Here's how the part is built. I have some questions about the finished solid (model axes, mm). A direction names the side the tool comes from. Coordinates: 2 decimals unless noted, no trailing zeros. Order: outer loops, then holes, each group sorted by start corner. A loop starts at its lowest first (then second) coordinate and runs counter-clockwise, first axis right, second up. Notation, with made-up numbers: (-39, 28.25) - (-19, 28.25) arc R22 cw to (-19, 46.25) - close; hole circle Ø3 at (-30.5, 21). An arc over 180 degrees is marked (long way). Answer as CSV lines item,"result". Start each with the question number.
Q1. For faces 4 (the face through (-1115, 734, -1921.897)), 5 (the face through (-1143, 746, -1943.397)), 6 (the face through (-1127.528, 743, -1930)), 7 (the face through (-1143, 740, -1917.397)), which set-ups out of +Z, -Z, +X, -X, +Y, -Y let a thin tool reach every point of the face, with its end or its side?
Q2. Thinking about a two-plate mould opening in X: for faces 1 (the face through (-1158.528, 746, -1930)), 2 (the face through (-1128, 732.908, -1929)), 3 (the face through (-1115, 734, -1936.897)), which applies, released by +X, released by -X, zero draft, split by the parting line, or undercut?
Q3. I need wall thicknesses on line 1 (X direction, y = 733.75, z = -1941.5); line 2 (X direction, y = 738.75, z = -1931); line 3 (Z direction, x = -1148.5, y = 729). Which ranges of each line are inside material? Lowest first, please.
Q4. Suppose I cut it at A-A (z = -1926.5). Please give me the cut outline in (x, y), then the cut area to 3 significant figures.
Q5. For pin 1 Ø10 at (y, z) = (731.5, -1931) entering from +X; pin 2 Ø13 at (y, z) = (746.5, -1933) entering from +X; pin 3 Ø4 at (x, y) = (-1151, 737) entering from +Z, each with a flat end and sliding along its axis, tell me the tip position at first contact or that it passes through.
Q6. Suppose I cut it at D-D (x = -1152.5). Please give me the cut outline in (y, z).
Q7. Suppose I cut it at B-B (x = -1121). Please give me the cut outline in (y, z).
Q8. Suppose I cut it at C-C (y = 736.5). Please give me the cut outline in (x, z), then the cut area to 3 significant figures.
from build123d import *

# Parameters (mm, degrees)
SKETCH3_W           = 4000
SKETCH3_H           = 4000
BOSS_EXTRUDE1_DEPTH = 1250
SKETCH4_W           = 3200
SKETCH4_H           = 2700
BOSS_EXTRUDE2_DEPTH = 1200
SKETCH6_W           = 3000
SKETCH6_H           = 2500
CUT_EXTRUDE1_DEPTH  = 6011.745093863
SKETCH9_W           = 2000
SKETCH9_H           = 690
BOSS_EXTRUDE8_DEPTH = 150
SKETCH8_W           = 2000
SKETCH8_H           = 690
BOSS_EXTRUDE9_DEPTH = 150
SKETCH13_W          = 1250
SKETCH13_H          = 1250
BOSS_EXTRUDE5_DEPTH = 1250
SKETCH14_W          = 1250
SKETCH14_H          = 1250
BOSS_EXTRUDE6_DEPTH = 1250
SCALE1_SCALE        = 0.01


with BuildPart() as part:
    # Sketch3 → Boss-Extrude1 (new body)
    with BuildSketch(Plane(origin=(0, 0, 0), x_dir=(1, 0, 0), z_dir=(0, 1, 0))):
        with Locations((-1806.81348539, 1954.077347606)):
            Rectangle(SKETCH3_W, SKETCH3_H)
    extrude(amount=BOSS_EXTRUDE1_DEPTH)

    # Sketch4 → Boss-Extrude2 (add)
    with BuildSketch(Plane(origin=(0, 1250, 0), x_dir=(1, 0, 0), z_dir=(0, 1, 0))):
        with Locations((-1900, 2000)):
            Rectangle(SKETCH4_W, SKETCH4_H)
    extrude(amount=BOSS_EXTRUDE2_DEPTH)

    # Sketch6 → Cut-Extrude1 (cut, through all)
    with BuildSketch(Plane(origin=(0, 2450, 0), x_dir=(1, 0, 0), z_dir=(0, 1, 0))):
        with Locations((-1900, 2000)):
            Rectangle(SKETCH6_W, SKETCH6_H)
    extrude(amount=-CUT_EXTRUDE1_DEPTH, mode=Mode.SUBTRACT)

    # Sketch9 → Boss-Extrude8 (add)
    with BuildSketch(Plane.ZY.offset(400)):
        with Locations((-1900, 900)):
            Rectangle(SKETCH9_W, SKETCH9_H)
    extrude(amount=BOSS_EXTRUDE8_DEPTH)

    # Sketch8 → Boss-Extrude9 (add)
    with BuildSketch(Plane(origin=(-3400, 0, 0), x_dir=(0, 0, -1), z_dir=(1, 0, 0))):
        with Locations((1900, 900)):
            Rectangle(SKETCH8_W, SKETCH8_H)
    extrude(amount=BOSS_EXTRUDE9_DEPTH)

    # Sketch13 → Boss-Extrude5 (add)
    with BuildSketch(Plane(origin=(193.18651461, 0, 0), x_dir=(0, 0, -1), z_dir=(1, 0, 0))):
        with Locations((575, 625)):
            Rectangle(SKETCH13_W, SKETCH13_H)
    extrude(amount=BOSS_EXTRUDE5_DEPTH)

    # Sketch14 → Boss-Extrude6 (add)
    with BuildSketch(Plane(origin=(193.18651461, 0, 0), x_dir=(0, 0, -1), z_dir=(1, 0, 0))):
        with Locations((3325, 625)):
            Rectangle(SKETCH14_W, SKETCH14_H)
    extrude(amount=BOSS_EXTRUDE6_DEPTH)


with BuildPart() as part_1:
    # Scale1: scaled about (-1134.876780231, 734.705300906, -1929.188509471)
    add(part.part.scale(SCALE1_SCALE).moved(Location((-1123.528012429, 727.358247897, -1909.896624376))))


solid = part_1.part
Here are the results:
1,face 4,"+X, +Y, -Y"
1,face 5,"-Z, +X, -X, +Y"
1,face 6,"none"
1,face 7,"+Y, -Y"
2,face 1,"released by -X"
2,face 2,"undercut"
2,face 3,"zero draft"
3,line 1,"x = -1161.6 to -1157.53, -1127.53 to -1109.1"
3,line 2,"x = -1161.6 to -1156.03, -1129.03 to -1121.6"
3,line 3,"z = -1949.44 to -1942.4, -1917.4 to -1909.44"
4,outline,"(-1161.6, 727.36) - (-1157.53, 727.36) - (-1157.53, 732.91) - (-1156.03, 732.91) - (-1156.03, 739.81) - (-1157.53, 739.81) - (-1157.53, 751.86) - (-1158.53, 751.86) - (-1158.53, 739.86) - (-1161.6, 739.86) - close; (-1129.03, 732.91) - (-1127.53, 732.91) - (-1127.53, 727.36) - (-1121.6, 727.36) - (-1121.6, 739.86) - (-1126.53, 739.86) - (-1126.53, 751.86) - (-1127.53, 751.86) - (-1127.53, 739.81) - (-1129.03, 739.81) - close"
4,area,"170 mm²"
5,pin 1,"stops at x = -1121.6"
5,pin 2,"stops at x = -1126.53"
5,pin 3,"stops at z = -1909.44"
6,outline,"(727.36, -1949.44) - (739.86, -1949.44) - (739.86, -1943.4) - (751.86, -1943.4) - (751.86, -1942.4) - (727.36, -1942.4) - close; (727.36, -1917.4) - (751.86, -1917.4) - (751.86, -1916.4) - (739.86, -1916.4) - (739.86, -1909.44) - (727.36, -1909.44) - close"
7,outline,"(727.36, -1949.4) - (739.86, -1949.4) - (739.86, -1936.9) - (727.36, -1936.9) - close; (727.36, -1921.9) - (739.86, -1921.9) - (739.86, -1909.4) - (727.36, -1909.4) - close"
8,outline,"(-1161.6, -1949.44) - (-1121.6, -1949.44) - (-1121.6, -1949.4) - (-1109.1, -1949.4) - (-1109.1, -1936.9) - (-1121.6, -1936.9) - (-1121.6, -1921.9) - (-1109.1, -1921.9) - (-1109.1, -1909.4) - (-1121.6, -1909.4) - (-1121.6, -1909.44) - (-1161.6, -1909.44) - close; hole (-1157.53, -1942.4) - (-1127.53, -1942.4) - (-1127.53, -1938.9) - (-1129.03, -1938.9) - (-1129.03, -1918.9) - (-1127.53, -1918.9) - (-1127.53, -1917.4) - (-1157.53, -1917.4) - (-1157.53, -1918.9) - (-1156.03, -1918.9) - (-1156.03, -1938.9) - (-1157.53, -1938.9) - close"
8,area,"1,220 mm²"
